```python
from build123d import *

# Parameters (mm, degrees)
BOSS_EXTRUDE1_DEPTH = 1020
SKETCH2_W           = 25
SKETCH2_H           = 25
CUT_EXTRUDE1_DEPTH  = 10
SKETCH3_R           = 3
CUT_EXTRUDE2_DEPTH  = 10
LPATTERN1_COUNT     = 9
LPATTERN1_PITCH     = 97


with BuildPart() as part:
    # Sketch1 → Boss-Extrude1 (new body)
    with BuildSketch(Plane.XY):
        Polygon((0, 10), (0, 0), (60, 0), (60, 10), (55, 10), (55, 5), (25, 5), (25, 95), (15, 95), (15, 5), (5, 5), (5, 10), align=None)
    extrude(amount=BOSS_EXTRUDE1_DEPTH)

    # Sketch2 → Cut-Extrude1 (cut)
    with BuildSketch(Plane(origin=(25, 0, 0), x_dir=(0, 0, -1), z_dir=(1, 0, 0))):
        with Locations((-1007.5, 82.5)):
            Rectangle(SKETCH2_W, SKETCH2_H)
        with Locations((-12.5, 82.5)):
            Rectangle(SKETCH2_W, SKETCH2_H)
    extrude(amount=-CUT_EXTRUDE1_DEPTH, mode=Mode.SUBTRACT)

    # Sketch3 → Cut-Extrude2 (cut)
    with BuildSketch(Plane(origin=(25, 0, 0), x_dir=(0, 0, -1), z_dir=(1, 0, 0))):
        with Locations(Location((-898, 85, 0), (0, 0, 90))):
            Circle(SKETCH3_R)
    cut_extrude2 = extrude(amount=-CUT_EXTRUDE2_DEPTH, mode=Mode.SUBTRACT)

    # LPattern1: Cut-Extrude2 ×9
    with Locations(*[(0, 0, -i * LPATTERN1_PITCH) for i in range(1, LPATTERN1_COUNT)]):
        add(cut_extrude2, mode=Mode.SUBTRACT)


solid = part.part
```
Geometry: final body of the model. Coordinates: model frame, mm. Round coordinates to 2 decimals unless told otherwise and drop trailing zeros. Order: outer loops, then holes, each group sorted by start corner. A loop starts at its lowest first (then second) coordinate and runs counter-clockwise, first axis right, second up. Notation, with made-up numbers: (-7, 77) -> (47, 77) arc R29 ccw to (47, 105) -> close; hole circle Ø8 at (32.5, 40.25). An arc over 180 degrees is marked (long way). Use one line per item in the form item = value. Start each with the question number.
1. Cut plane B-B (y = 58). Return the cut outline in (x, z), then the cut area to 3 significant figures.
2. Draft query along X for faces 1 (the face through (30, 0, 503)), 2 (the face through (40, 5, 503)). Return one class per face: pulls with the +X half, pulls with the -X half, needs draft (parallel to the pull), parting line crosses it, or undercut.
3. Cut plane C-C (x = 34). Return the cut outline in (y, z), then the cut area to 3 significant figures.
4. Pin query (flat end, axial travel): pin 1 Ø10 at (y, z) = (66.5, 291) entering from -X; pin 2 Ø5.5 at (x, z) = (3.5, 522.5) entering from +Y; pin 3 Ø2 at (y, z) = (23, 785.5) entering from +X; pin 4 Ø5 at (y, z) = (85, 607) entering from -X. Return the tip coordinate at first contact, or that it passes through.
5. Line query: probe 1 along X at (y, z) = (8, 859); probe 2 along Y at (x, z) = (23, 122); probe 3 along Y at (x, z) = (5.5, 514.5). Output: solid intervals per line, ascending.
6. Cut plane A-A (z = 762.5). Return the cut outline in (x, y), then the cut area to 3 significant figures.
Solution:
q1.outline = (15, 0) -> (25, 0) -> (25, 1020) -> (15, 1020) -> close
q1.area = 10,200 mm^2
q2.face_1 = needs draft
q2.face_2 = undercut
q3.outline = (0, 0) -> (5, 0) -> (5, 1020) -> (0, 1020) -> close
q3.area = 5,100 mm^2
q4.pin_1 = 15
q4.pin_2 = 10
q4.pin_3 = 25
q4.pin_4 = through
q5.probe_1 = 0 to 5, 15 to 25, 55 to 60
q5.probe_2 = 0 to 82, 88 to 95
q5.probe_3 = 0 to 5
q6.outline = (0, 0) -> (60, 0) -> (60, 10) -> (55, 10) -> (55, 5) -> (25, 5) -> (25, 95) -> (15, 95) -> (15, 5) -> (5, 5) -> (5, 10) -> (0, 10) -> close
q6.area = 1,250 mm^2
